Input: part model. Units: mm. Frame: model coordinates. Coordinates: 2 decimals unless noted, no trailing zeros. Write each loop counter-clockwise with the first axis right and the second up, starting at its lowest first coordinate (ties: lowest second). Pieces come first, ordered by that corner, then holes.
from build123d import *

# Parameters (mm, degrees)
F1_DEPTH     = 7.5
F1_TAPER     = 30
F2_R         = 3
F3_DEPTH     = 15.0010001
F4_T1_DEPTH  = 17.3205080757
F4_T3_DEPTH  = 12.3205080757
F4_T5_DEPTH  = 17.3205080757
F4_T7_DEPTH  = 12.3205080757
F4_T9_DEPTH  = 12.3205080757
F4_T11_DEPTH = 12.3205080757
F4_T13_DEPTH = 12.3205080757
F4_T15_DEPTH = 17.3205080757
F4_T17_DEPTH = 17.3205080757
F4_T19_DEPTH = 17.3205080757


# Not quite as in the source:
# - a fillet or chamfer that OpenCascade refuses, or shapes differently, is made with other operations: its cross-section is extruded or revolved along the edge and cut away or added


with BuildPart() as f1:
    # F0 (on Top) → F1 (new body, symmetric)
    with BuildSketch(Plane.XY):
        Polygon((10, -5.7735026919), (10, 5.7735026919), (0, 11.5470053838), (-10, 5.7735026919), (-10, -5.7735026919), (0, -11.5470053838), align=None)
    extrude(amount=F1_DEPTH, both=True, taper=F1_TAPER)

    # F2 (on face) → F3 (cut, through all)
    with BuildSketch(Plane.XY.offset(7.5)):
        Circle(F2_R)
    extrude(amount=-F3_DEPTH, mode=Mode.SUBTRACT)

    # F4: fillet of radius 2 on 21 edges, made by hand

    # F4_s2 → F4_t1 (cut)
    with BuildSketch(Plane.XZ.offset(-8.6602540378)):
        with BuildLine():
            ThreePointArc((9.4226497308, -1), (9.6905989232, 0), (9.4226497308, 1))
            Line((9.4226497308, 1), (10, 0))
            Line((10, 0), (9.4226497308, -1))
        make_face()
        with BuildLine():
            ThreePointArc((-9.4226497308, -1), (-9.6905989232, 0), (-9.4226497308, 1))
            Line((-9.4226497308, 1), (-10, 0))
            Line((-10, 0), (-9.4226497308, -1))
        make_face()
    extrude(amount=F4_T1_DEPTH, mode=Mode.SUBTRACT)

    # F4_s4 → F4_t3 (cut)
    with BuildSketch(Plane.XZ.offset(-6.1602540378)):
        with BuildLine():
            ThreePointArc((6.2472232503, -6.5), (5.5151724427, -7.2320508076), (4.5151724427, -7.5))
            Line((4.5151724427, -7.5), (5.6698729811, -7.5))
            Line((5.6698729811, -7.5), (6.2472232503, -6.5))
        make_face()
        with BuildLine():
            ThreePointArc((6.2472232503, 6.5), (5.5151724427, 7.2320508076), (4.5151724427, 7.5))
            Line((4.5151724427, 7.5), (5.6698729811, 7.5))
            Line((5.6698729811, 7.5), (6.2472232503, 6.5))
        make_face()
        with BuildLine():
            ThreePointArc((-4.5151724427, -7.5), (-5.5151724427, -7.2320508076), (-6.2472232503, -6.5))
            Line((-6.2472232503, -6.5), (-5.6698729811, -7.5))
            Line((-5.6698729811, -7.5), (-4.5151724427, -7.5))
        make_face()
        with BuildLine():
            ThreePointArc((-4.5151724427, 7.5), (-5.5151724427, 7.2320508076), (-6.2472232503, 6.5))
            Line((-6.2472232503, 6.5), (-5.6698729811, 7.5))
            Line((-5.6698729811, 7.5), (-4.5151724427, 7.5))
        make_face()
    extrude(amount=F4_T3_DEPTH, mode=Mode.SUBTRACT)

    # F4_s6 → F4_t5 (cut)
    with BuildSketch(Plane(origin=(7.5, -4.3301270189, 0), x_dir=(0, 0, 1), z_dir=(-0.8660254038, 0.5, 0))):
        with BuildLine():
            ThreePointArc((-1, 9.4226497308), (0, 9.6905989232), (1, 9.4226497308))
            Line((1, 9.4226497308), (0, 10))
            Line((0, 10), (-1, 9.4226497308))
        make_face()
    extrude(amount=F4_T5_DEPTH, mode=Mode.SUBTRACT)

    # F4_s8 → F4_t7 (cut)
    with BuildSketch(Plane(origin=(5.3349364905, -3.0801270189, 0), x_dir=(0, 0, 1), z_dir=(-0.8660254038, 0.5, 0))):
        with BuildLine():
            ThreePointArc((-6.5, 6.2472232503), (-7.2320508076, 5.5151724427), (-7.5, 4.5151724427))
            Line((-7.5, 4.5151724427), (-7.5, 5.6698729811))
            Line((-7.5, 5.6698729811), (-6.5, 6.2472232503))
        make_face()
        with BuildLine():
            ThreePointArc((6.5, 6.2472232503), (7.2320508076, 5.5151724427), (7.5, 4.5151724427))
            Line((7.5, 4.5151724427), (7.5, 5.6698729811))
            Line((7.5, 5.6698729811), (6.5, 6.2472232503))
        make_face()
    extrude(amount=F4_T7_DEPTH, mode=Mode.SUBTRACT)

    # F4_s10 → F4_t9 (cut)
    with BuildSketch(Plane(origin=(-5.3349364905, -3.0801270189, 0), x_dir=(0, 0, 1), z_dir=(0.8660254038, 0.5, 0))):
        with BuildLine():
            ThreePointArc((-7.5, 4.5151724427), (-7.2320508076, 5.5151724427), (-6.5, 6.2472232503))
            Line((-6.5, 6.2472232503), (-7.5, 5.6698729811))
            Line((-7.5, 5.6698729811), (-7.5, 4.5151724427))
        make_face()
        with BuildLine():
            ThreePointArc((6.5, 6.2472232503), (7.2320508076, 5.5151724427), (7.5, 4.5151724427))
            Line((7.5, 4.5151724427), (7.5, 5.6698729811))
            Line((7.5, 5.6698729811), (6.5, 6.2472232503))
        make_face()
    extrude(amount=F4_T9_DEPTH, mode=Mode.SUBTRACT)

    # F4_s12 → F4_t11 (cut)
    with BuildSketch(Plane(origin=(-5.3349364905, 3.0801270189, 0), x_dir=(0, 0, 1), z_dir=(0.8660254038, -0.5, 0))):
        with BuildLine():
            ThreePointArc((-7.5, 4.5151724427), (-7.2320508076, 5.5151724427), (-6.5, 6.2472232503))
            Line((-6.5, 6.2472232503), (-7.5, 5.6698729811))
            Line((-7.5, 5.6698729811), (-7.5, 4.5151724427))
        make_face()
        with BuildLine():
            ThreePointArc((7.5, 4.5151724427), (7.2320508076, 5.5151724427), (6.5, 6.2472232503))
            Line((6.5, 6.2472232503), (7.5, 5.6698729811))
            Line((7.5, 5.6698729811), (7.5, 4.5151724427))
        make_face()
    extrude(amount=F4_T11_DEPTH, mode=Mode.SUBTRACT)

    # F4_s14 → F4_t13 (cut)
    with BuildSketch(Plane(origin=(5.3349364905, 3.0801270189, 0), x_dir=(0, 0, 1), z_dir=(-0.8660254038, -0.5, 0))):
        with BuildLine():
            ThreePointArc((-7.5, 4.5151724427), (-7.2320508076, 5.5151724427), (-6.5, 6.2472232503))
            Line((-6.5, 6.2472232503), (-7.5, 5.6698729811))
            Line((-7.5, 5.6698729811), (-7.5, 4.5151724427))
        make_face()
        with BuildLine():
            ThreePointArc((7.5, 4.5151724427), (7.2320508076, 5.5151724427), (6.5, 6.2472232503))
            Line((6.5, 6.2472232503), (7.5, 5.6698729811))
            Line((7.5, 5.6698729811), (7.5, 4.5151724427))
        make_face()
    extrude(amount=F4_T13_DEPTH, mode=Mode.SUBTRACT)

    # F4_s16 → F4_t15 (cut)
    with BuildSketch(Plane(origin=(-7.5, -4.3301270189, 0), x_dir=(0, 0, 1), z_dir=(0.8660254038, 0.5, 0))):
        with BuildLine():
            ThreePointArc((-1, 9.4226497308), (0, 9.6905989232), (1, 9.4226497308))
            Line((1, 9.4226497308), (0, 10))
            Line((0, 10), (-1, 9.4226497308))
        make_face()
    extrude(amount=F4_T15_DEPTH, mode=Mode.SUBTRACT)

    # F4_s18 → F4_t17 (cut)
    with BuildSketch(Plane(origin=(7.5, 4.3301270189, 0), x_dir=(0, 0, 1), z_dir=(-0.8660254038, -0.5, 0))):
        with BuildLine():
            ThreePointArc((-1, 9.4226497308), (0, 9.6905989232), (1, 9.4226497308))
            Line((1, 9.4226497308), (0, 10))
            Line((0, 10), (-1, 9.4226497308))
        make_face()
    extrude(amount=F4_T17_DEPTH, mode=Mode.SUBTRACT)

    # F4_s20 → F4_t19 (cut)
    with BuildSketch(Plane(origin=(-7.5, 4.3301270189, 0), x_dir=(0, 0, 1), z_dir=(0.8660254038, -0.5, 0))):
        with BuildLine():
            ThreePointArc((-1, 9.4226497308), (0, 9.6905989232), (1, 9.4226497308))
            Line((1, 9.4226497308), (0, 10))
            Line((0, 10), (-1, 9.4226497308))
        make_face()
    extrude(amount=F4_T19_DEPTH, mode=Mode.SUBTRACT)

    # F4_s21 → F4_t22 (revolve, cut)
    with BuildSketch(Plane.XZ):
        with BuildLine():
            ThreePointArc((5, -7.5), (3.5857864376, -6.9142135624), (3, -5.5))
            Line((3, -5.5), (3, -7.5))
            Line((3, -7.5), (5, -7.5))
        make_face()
    revolve(axis=Axis((0, 0, -7.5), (0, 0, 1)), mode=Mode.SUBTRACT)

    # F4_s23 → F4_t24 (revolve, cut)
    with BuildSketch(Plane.XZ):
        with BuildLine():
            ThreePointArc((5, 7.5), (3.5857864376, 6.9142135624), (3, 5.5))
            Line((3, 5.5), (3, 7.5))
            Line((3, 7.5), (5, 7.5))
        make_face()
    revolve(axis=Axis((0, 0, 7.5), (0, 0, 1)), mode=Mode.SUBTRACT)


solid = f1.part
Item 1: Pin query (flat end, axial travel): pin 1 Ø1.5 at (x, z) = (4.5, 2.5) entering from +Y; pin 2 Ø5 at (x, z) = (4.5, 2) entering from -Y; pin 3 Ø2 at (x, y) = (2, -8) entering from +Z; pin 4 Ø5 at (x, y) = (0, 0) entering from -Z. Return the tip coordinate at first contact, or that it passes through.
Item 2: Section query A-A, the plane z = 4.75. Return loops of the section in (x, y).
Item 3: Material intervals for line 1 (Y direction, x = -8, z = -0.5); line 2 (Y direction, x = -1, z = 5); line 3 (Y direction, x = 1.75, z = -3.75), sorted ascending.
The answers:
1. pin 1: stops at y = 7.94
1. pin 2: stops at y = -9.68
1. pin 3: stops at z = 5.32
1. pin 4: passes through
2. outline: (-7.26, -4.19) - (0, -8.38) - (7.26, -4.19) - (7.26, 4.19) - (0, 8.38) - (-7.26, 4.19) - close; hole circle Ø6 at (0, 0)
3. line 1: y = -6.5 to 6.5
3. line 2: y = -7.64 to -2.83, 2.83 to 7.64
3. line 3: y = -8.04 to -2.44, 2.44 to 8.04
